```python
from build123d import *

# Parameters (mm, degrees)
BOSS_EXTRUDE1_START = -4
BOSS_EXTRUDE1_DEPTH = 8
SKETCH4_R           = 20
SKETCH4_R_2         = 12.5
SKETCH4_R_3         = 25
BOSS_EXTRUDE5_DEPTH = 10


# Read off the part's stored shape, not the designer's step: Boss-Extrude1
with BuildPart() as part:
    # Boss-Extrude1 outline → Boss-Extrude1 (new body)
    with BuildSketch(Plane.XY.offset(BOSS_EXTRUDE1_START)):
        with BuildLine():
            add(Edge.make_bspline(
                [(3.005567425, 19.772874461), (18.916222227, 17.720110762), (215.876421889, 18.298562521), (231.273379323, 23.427464471)],
                knots=[0.02790249, 0.02790249, 0.02790249, 0.02790249, 0.919000917, 0.919000917, 0.919000917, 0.919000917], degree=3))
            ThreePointArc((3.005567425, 19.772874461), (19.964927421, 1.183922747), (5.321353729, -19.279086973))
            add(Edge.make_bspline(
                [(5.321353729, -19.279086973), (29.380163277, -15.107768003), (216.311047881, -18.024838758), (231.401749268, -23.474881988)],
                knots=[0.059243279, 0.059243279, 0.059243279, 0.059243279, 0.920155583, 0.920155583, 0.920155583, 0.920155583], degree=3))
            ThreePointArc((231.401749268, -23.474881988), (215.000093636, -0.068423797), (231.273379323, 23.427464471))
        make_face()
    extrude(amount=BOSS_EXTRUDE1_DEPTH)

    # Sketch4 → Boss-Extrude5 (add, symmetric)
    # profile 1 of 2: a face of its own
    with BuildSketch(Plane.XY):
        Circle(SKETCH4_R)
        Circle(SKETCH4_R_2, mode=Mode.SUBTRACT)
    # profile 2 of 2: a face of its own
    with BuildSketch(Plane.XY):
        with Locations((240, 0)):
            Circle(SKETCH4_R_3)
        with Locations((240, 0)):
            Circle(SKETCH4_R_2, mode=Mode.SUBTRACT)
    extrude(amount=BOSS_EXTRUDE5_DEPTH, both=True)


solid = part.part
```
Can you work these out from the model? Positions are in its coordinate system, mm. A direction names the side the tool comes from. Give positions to 0.01 mm unless a question says otherwise; leave off trailing zeros. Write each loop counter-clockwise with the first axis right and the second up, starting at its lowest first coordinate (ties: lowest second). Pieces come first, ordered by that corner, then holes. Notation, with made-up numbers: (31, -3.75) -> (48, -3.75) arc R20 ccw to (48, 19.25) -> close; hole circle Ø5 at (54.25, 8.5). An arc over 180 degrees is marked (long way). Write item = value, one per line.
(1) I need wall thicknesses on probe 1 along X at (y, z) = (1, 5.25); probe 2 along X at (y, z) = (9.5, 0.5); probe 3 along Y at (x, z) = (240, 5). Which ranges of each line are inside material? Lowest first, please. Write a range as from..to.
Worked out:
probe_1 = -19.97..-12.46, 12.46..19.97, 215.02..227.54, 252.46..264.98
probe_2 = -17.6..-8.12, 8.12..231.88, 248.12..263.12
probe_3 = -25..-12.5, 12.5..25
(2) Suppose I cut it at A-A on y = 0. Write out the boundary of the cut face in (x, z), then the cut area to 3 significant figures.
Worked out:
outline = (-20, -10) -> (-12.5, -10) -> (-12.5, 10) -> (-20, 10) -> close; (12.5, -10) -> (20, -10) -> (20, -4) -> (215, -4) -> (215, -10) -> (227.5, -10) -> (227.5, 10) -> (215, 10) -> (215, 4) -> (20, 4) -> (20, 10) -> (12.5, 10) -> close; (252.5, -10) -> (265, -10) -> (265, 10) -> (252.5, 10) -> close
area = 2,360 mm^2
(3) Thinking about a two-plate mould opening in X: for faces 3 (the face through (119, 0, 4)), 4 (the face through (9, 9, -10)), which applies, released by +X, released by -X, zero draft, split by the parting line, or undercut?
Worked out:
face_3 = undercut
face_4 = zero draft
(4) Suppose I cut it at B-B on x = 240. Write out the boundary of the cut face in (y, z).
Worked out:
outline = (-25, -10) -> (-12.5, -10) -> (-12.5, 10) -> (-25, 10) -> close; (12.5, -10) -> (25, -10) -> (25, 10) -> (12.5, 10) -> close
(5) For faces 1 (the face through (263.846, 7.509, 0.14)), 2 (the face through (251.923, 3.755, -0.14)), which set-ups out of +Z, -Z, +X, -X, +Y, -Y let a thin tool reach every point of the face, with its end or its side?
Worked out:
face_1 = none
face_2 = +Z, -Z
(6) I'm going to push flat-ended pins straight in: P1, Ø1.5, axis at y = 6, z = -3, coming from the +X side; P2, Ø6, axis at x = 211.5, z = 6, coming from the -Y side; P3, Ø20, axis at x = 0, y = 0, coming from the +Z side; P4, Ø1.5, axis at x = 181.5, y = -0.5, coming from the +Z side. Where does each tip first touch, or does it pass through?
Worked out:
P1 = 264.44
P2 = -21.18
P3 = through
P4 = 4
(7) Suppose I cut it at C-C on z = -6.75. Write out the boundary of the cut face in (x, y), then the cut area to 3 significant figures.
Worked out:
outline = circle Ø40 at (0, 0); circle Ø50 at (240, 0); hole circle Ø25 at (0, 0); hole circle Ø25 at (240, 0)
area = 2,240 mm^2
